Build history of the part. All positions in model axes, mm. Face numbers are marked on the shaded views. A direction names the side the tool comes from. Give positions to 0.01 mm unless a question says otherwise; leave off trailing zeros. Write each loop counter-clockwise with the first axis right and the second up, starting at its lowest first coordinate (ties: lowest second). Pieces come first, ordered by that corner, then holes. Notation, with made-up numbers: (38.5, -17.75) -> (63.5, -17.75) arc R27 ccw to (63.5, 1.25) -> close; hole circle Ø6 at (34.25, -11.5). An arc over 180 degrees is marked (long way). Put each result on its own line as item: value. Start each with the question number.
Item 1: Slice it at A-A, the plane z = 11.6. List the corners of the cut face in (x, y), plus the area to 3 significant figures.
Item 2: Drill centre lines: line 1 along Z through (x, y) = (-29.4, -40); line 2 along Y through (x, z) = (13.5, -2.5); line 3 along Z through (x, y) = (0, -2.5). Where is each one in solid material? Low to high.
Item 3: Flat gauge pins, fed straight in: pin 1 Ø5 at (x, z) = (-13.5, 0) entering from -Y; pin 2 Ø6 at (y, z) = (-30.5, 2) entering from +X; pin 3 Ø4 at (x, z) = (-28.5, 10.5) entering from +Y. Where does each tip first touch, or does it go through?
Item 4: Slice it at C-C, the plane x = -13.5. List the corners of the cut face in (y, z), plus the area to 3 significant figures.
Item 5: Tool access for the marked faces 1, 2 and 3: list every direction of +Z, -Z, +X, -X, +Y, -Y with a clear straight run to the whole face (end or side of a thin tool).
Item 6: Slice it at D-D, the plane y = -27.5. List the corners of the cut face in (x, z), plus the area to 3 significant figures.
Item 7: Slice it at B-B, the plane y = -40. List the corners of the cut face in (x, z), plus the area to 3 significant figures.
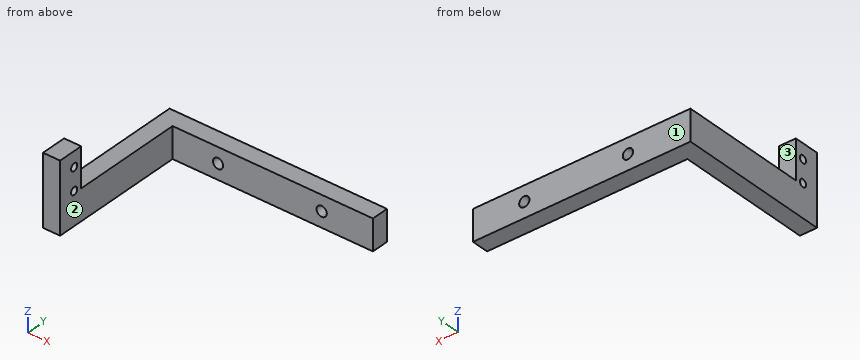
```python
from build123d import *

# Parameters (mm, degrees)
F0_W     = 63.6
F0_H     = 9
F0_R     = 1.5
F1_DEPTH = 5
F2_W     = 5
F2_H     = 9
F3_DEPTH = 40
F4_W     = 5
F4_H     = 7.5
F5_DEPTH = 11.5
F6_R     = 1.1
F7_DEPTH = 5.001


with BuildPart() as f1:
    # F0 (on Front) → F1 (new body)
    with BuildSketch(Plane.XZ):
        Rectangle(F0_W, F0_H)
        with Locations((-13.5, 0)):
            Circle(F0_R, mode=Mode.SUBTRACT)
        with Locations((16.8, 0)):
            Circle(F0_R, mode=Mode.SUBTRACT)
    extrude(amount=F1_DEPTH)

    # F2 (on face) → F3 (join)
    with BuildSketch(Plane.XZ.offset(5)):
        with Locations((-29.3, 0)):
            Rectangle(F2_W, F2_H)
    extrude(amount=F3_DEPTH)

    # F4 (on face) → F5 (join)
    with BuildSketch(Plane.XY.offset(4.5)):
        with Locations((-29.3, -41.25)):
            Rectangle(F4_W, F4_H)
    extrude(amount=F5_DEPTH)

    # F6 (on face) → F7 (cut, through all)
    with BuildSketch(Plane.YZ.offset(-26.8)):
        with Locations((-40, 5.1)):
            Circle(F6_R)
        with Locations((-40, 11.6)):
            Circle(F6_R)
    extrude(amount=-F7_DEPTH, mode=Mode.SUBTRACT)


solid = f1.part
```
Values follow:
1. outline: (-31.8, -45) -> (-26.8, -45) -> (-26.8, -41.1) -> (-31.8, -41.1) -> close; (-31.8, -38.9) -> (-26.8, -38.9) -> (-26.8, -37.5) -> (-31.8, -37.5) -> close
1. area: 26.5 mm2
2. line 1: -4.5 to 4, 6.2 to 10.5, 12.7 to 16
2. line 2: -5 to 0
2. line 3: -4.5 to 4.5
3. pin 1: y = -5
3. pin 2: x = -26.8
3. pin 3: y = -37.5
4. outline: (-5, -4.5) -> (0, -4.5) -> (0, -1.5) -> (-5, -1.5) -> close; (-5, 1.5) -> (0, 1.5) -> (0, 4.5) -> (-5, 4.5) -> close
4. area: 30.0 mm2
5. face 1: +Z, -Z, +X, -X, +Y
5. face 2: +Z, -Z, +X, -Y
5. face 3: +Z, +X, -X, +Y
6. outline: (-31.8, -4.5) -> (-26.8, -4.5) -> (-26.8, 4.5) -> (-31.8, 4.5) -> close
6. area: 45.0 mm2
7. outline: (-31.8, -4.5) -> (-26.8, -4.5) -> (-26.8, 4) -> (-31.8, 4) -> close; (-31.8, 6.2) -> (-26.8, 6.2) -> (-26.8, 10.5) -> (-31.8, 10.5) -> close; (-31.8, 12.7) -> (-26.8, 12.7) -> (-26.8, 16) -> (-31.8, 16) -> close
7. area: 80.5 mm2
